from build123d import *

# Parameters (mm, degrees)
ESQUISSE1_R        = 1.6
BOSS_EXTRU_1_DEPTH = 3


with BuildPart() as part:
    # Esquisse1 → Boss.-Extru.1 (new body)
    with BuildSketch(Plane.XY):
        Polygon((-130.649820486, -22.415487094), (-119.070790786, -62.796362516), (-120.442039466, -65.27016062), (-138.268849115, -70.381916029), (-140.742647218, -69.010667349), (-154.419403971, -21.314148304), (-165.848732708, -12.701531345), (-206.165691337, -12.701531345), (-221.686141291, -8.251113935), (-228.411595336, -6.322621021), (-237.526398495, -3.709541892), (-245.374022141, -1.459744369), (-249.872259625, -3.248768002), (-288.323340616, 7.774587685), (-291.190458161, 11.675149567), (-324.146226634, 21.123080509), (-329.606279511, 18.096325283), (-352.324375235, -61.131089881), (-349.297882974, -66.591026451), (-293.334748244, -82.638197107), (-287.498708924, -98.561018129), (-250.280154874, -115.48724507), (-232.892593163, -133.444615579), (-226.653475651, -133.542771169), (-198.570548361, -106.350948678), (-137.019971382, -106.350948678), (-108.937044092, -133.542771169), (-102.69792658, -133.444615579), (-85.310364869, -115.48724507), (-48.091810819, -98.561018129), (-42.255771499, -82.638197107), (13.707363231, -66.591026451), (16.733855492, -61.131089881), (-5.984240232, 18.096325283), (-11.444293109, 21.123080509), (-44.400061582, 11.675149567), (-47.267179127, 7.774587685), (-85.718260118, -3.248768002), (-90.216497602, -1.459744369), (-98.064121248, -3.709541892), (-107.178924407, -6.322621021), (-113.904378452, -8.251113935), (-124.479201425, -11.283395628), align=None)
        with Locations((-229.666591606, -126.713325795)):
            Circle(ESQUISSE1_R, mode=Mode.SUBTRACT)
        with Locations((-204.059552706, -101.880200807)):
            Circle(ESQUISSE1_R, mode=Mode.SUBTRACT)
        with Locations((-281.934339477, -93.401689518)):
            Circle(ESQUISSE1_R, mode=Mode.SUBTRACT)
        with Locations((-344.882804027, -60.574933915)):
            Circle(ESQUISSE1_R, mode=Mode.SUBTRACT)
        Polygon((-210.232188047, -30.001147656), (-224.390430785, -79.377961929), (-208.212806214, -96.161100182), (-207.491865187, -96.85509979), (-208.236606037, -97.572971364), (-229.533063287, -118.225792128), (-242.655085998, -104.673746846), (-258.969310369, -95.012679745), (-277.629290011, -88.825419148), (-272.289144354, -70.202118055), (-298.538981418, -62.6750984), (-299.849714513, -67.246167925), (-337.461409717, -56.461187875), (-321.404434006, -0.463858857), (-284.873898651, -10.938821309), (-283.564528345, -6.372504389), (-265.299260667, -11.609985616), (-264.679553884, -9.448811229), (-245.452786066, -14.960840928), (-246.072799476, -17.123084647), (-227.807531798, -22.360565873), (-228.496674065, -24.763890567), align=None, mode=Mode.SUBTRACT)
        Polygon((-187.078341197, -46.443029785), (-197.274945207, -82.010279702), (-199.748667041, -83.381665967), (-218.012930512, -78.145572016), (-219.384316777, -75.671850182), (-209.187712767, -40.104600265), (-206.713990933, -38.733214), (-188.449727462, -43.969307951), align=None, mode=Mode.SUBTRACT)
        with Locations((-105.923928137, -126.713325795)):
            Circle(ESQUISSE1_R, mode=Mode.SUBTRACT)
        with Locations((-131.530967037, -101.880200807)):
            Circle(ESQUISSE1_R, mode=Mode.SUBTRACT)
        with Locations((-53.656180266, -93.401689518)):
            Circle(ESQUISSE1_R, mode=Mode.SUBTRACT)
        Polygon((-106.057456456, -118.225792128), (-128.0696158, -96.878899722), (-127.377713529, -96.161100182), (-111.200088958, -79.377961929), (-125.358331696, -30.001147656), (-107.093845678, -24.763890567), (-107.782987945, -22.360565873), (-89.517720268, -17.123084647), (-90.137733677, -14.960840928), (-70.910965859, -9.448811229), (-70.291259076, -11.609985616), (-52.025991399, -6.372504389), (-50.716621092, -10.938821309), (-14.186085737, -0.463858857), (1.870889973, -56.461187875), (-35.740805231, -67.246167925), (-37.051538325, -62.6750984), (-63.301375389, -70.202118055), (-57.961229733, -88.825419148), (-76.621209374, -95.012679745), (-92.935433745, -104.673746846), align=None, mode=Mode.SUBTRACT)
        with Locations((9.292284284, -60.574933915)):
            Circle(ESQUISSE1_R, mode=Mode.SUBTRACT)
        with Locations((-167.795259872, -27.605548894)):
            Circle(ESQUISSE1_R, mode=Mode.SUBTRACT)
        with Locations((-323.590068827, 13.68165837)):
            Circle(ESQUISSE1_R, mode=Mode.SUBTRACT)
        with Locations((-216.832585966, -16.924131519)):
            Circle(ESQUISSE1_R, mode=Mode.SUBTRACT)
        with Locations((-118.757933777, -16.924131519)):
            Circle(ESQUISSE1_R, mode=Mode.SUBTRACT)
        with Locations((-12.000450916, 13.68165837)):
            Circle(ESQUISSE1_R, mode=Mode.SUBTRACT)
    extrude(amount=BOSS_EXTRU_1_DEPTH)


solid = part.part
For this review, take the finished solid that the model builds, in its own axes (mm). A direction names the side the tool comes from. Give positions to 0.01 mm unless a question says otherwise; leave off trailing zeros. Loops run counter-clockwise (first coordinate to the right, second up) from the corner with the lowest first, then second, coordinate; pieces in that order, holes last. Notation, with made-up numbers: (81.25, 64.25) -> (89.25, 64.25) arc R15 ccw to (89.25, 69.25) -> close; hole circle Ø8 at (66, 64.5). An arc over 180 degrees is marked (long way). One line per question, with ' | ' between items.
1) To check wall thickness, follow probe 1 along X at (y, z) = (-102, 0.6); probe 2 along Y at (x, z) = (-229, 1); probe 3 along Y at (x, z) = (-187, 2.05). State the ranges of each line that lie inside material, in increasing order.
Resolved:
probe 1: x = -279.94 to -247.17, -212.8 to -205.66, -202.46 to -133.13, -129.94 to -122.79, -88.42 to -55.65 | probe 2: y = -133.51 to -128.17, -125.26 to -117.71, -22.02 to -6.15 | probe 3: y = -106.35 to -12.7
2) Insertion check: pin 1 Ø3 at (x, y) = (-53.66, -93.4) entering from -Z (3 decimals); pin 2 Ø0.9 at (x, z) = (-160.5, 1) entering from -Y. Each pin has a flat end and moves straight along its axis. Give the tip position at first contact, or say it passes through.
Resolved:
pin 1: passes through | pin 2: stops at y = -106.35
3) We need section B-B (y = -110.5). Write out the cut boundary in (x, z).
Resolved:
outline: (-261.25, 0) -> (-237.01, 0) -> (-237.01, 3) -> (-261.25, 3) -> close; (-221.57, 0) -> (-202.86, 0) -> (-202.86, 3) -> (-221.57, 3) -> close; (-132.73, 0) -> (-114.02, 0) -> (-114.02, 3) -> (-132.73, 3) -> close; (-98.58, 0) -> (-74.34, 0) -> (-74.34, 3) -> (-98.58, 3) -> close
4) The part is to be moulded in two halves that separate along Y. For faces 1 (the flat face through (-241.71, -124.34, 1.48)), 2 (the flat face through (-124.941, -42.323, 1.479)), 3 (the flat face through (-307.438, 16.333, 1.479)), say which applies: +Y half, -Y half, draft (parallel to the pull), parting line (faces both ways), or undercut.
Resolved:
face 1: -Y half | face 2: undercut | face 3: +Y half
5) For faces 4 (the flat face through (-27.691, 16.465, 1.479)), 5 (the flat face through (-236.002, -111.545, 1.479)), 6 (the flat face through (-212.81, -120.14, 1.48)), list the 3-axis set-ups (+Z, -Z, +X, -X, +Y, -Y) from which the entire face can be reached by the end or side of a thin tool; tool diameter is ignored.
Resolved:
face 4: +Z, -Z, +Y | face 5: +Z, -Z | face 6: +Z, -Z, -Y
6) We need section A-A (x = -304). Write out the cut boundary in (y, z).
Resolved:
outline: (-79.58, 0) -> (-66.06, 0) -> (-66.06, 3) -> (-79.58, 3) -> close; (-5.45, 0) -> (15.35, 0) -> (15.35, 3) -> (-5.45, 3) -> close
7) We need section C-C (y = -35.5). Write out the cut boundary in (x, z), plus the area to 3 significant figures.
Resolved:
outline: (-344.97, 0) -> (-331.45, 0) -> (-331.45, 3) -> (-344.97, 3) -> close; (-211.81, 0) -> (-150.35, 0) -> (-150.35, 3) -> (-211.81, 3) -> close; (-126.9, 0) -> (-123.78, 0) -> (-123.78, 3) -> (-126.9, 3) -> close; (-4.14, 0) -> (9.38, 0) -> (9.38, 3) -> (-4.14, 3) -> close | area: 275 mm2
8) We need section D-D (z = 0.95). Give the number of separate pieces and of enclosed holes in the cut face, plus the area to 3 significant figures.
Resolved:
separate pieces: 1 | enclosed holes: 16 | area: 17,100 mm2
